Model file for the job. Use its own axes, mm. Face numbers are marked on the shaded views. A direction names the side the tool comes from. Round coordinates to 2 decimals unless told otherwise and drop trailing zeros. Order: outer loops, then holes, each group sorted by start corner. A loop starts at its lowest first (then second) coordinate and runs counter-clockwise, first axis right, second up. Notation, with made-up numbers: M 17,-28 L 48,-28 A38 cw 48,10 Z; hole C -10,35.5 d11. An arc over 180 degrees is marked long. Return JSON: item names as keys, results as strings. Group by question number.
Item 1: Pull direction Y, two halves, no side cores. Call the marked faces 4, 5 and 6: pulls with the +Y half, pulls with the -Y half, needs draft (parallel to the pull), parting line crosses it, or undercut.
Item 2: Slice it at B-B on z = 0. Write the cut outline in (x, y) (3 decimals).
Item 3: Which spindle directions (+Z, -Z, +X, -X, +Y, -Y) get a long thin tool onto all of the face, cutting with end or side? Do the marked faces 1, 2 and 3. Say none if no direction does.
Item 4: Pin check, flat tips, straight feed: pin 1 Ø3 at (y, z) = (9.5, -1) entering from +X; pin 2 Ø8 at (y, z) = (14.5, -4) entering from -X (3 decimals); pin 3 Ø5 at (y, z) = (12.5, -4.5) entering from +X; pin 4 Ø1.5 at (y, z) = (8, -1) entering from -X. Stop position of each tip, or through.
Item 5: Slice it at D-D on z = 3.5. Write the cut outline in (x, y).
Item 6: Slice it at C-C on y = 2. Write the cut outline in (x, z), then the cut area to 3 significant figures.
Item 7: Probe line 1 along Y through (x, z) = (-6.75, -5.75); line 2 along X through (y, z) = (7.75, 0). List the from-to ranges inside material, lowest first.
Item 8: Slice it at A-A on x = 0. Write the cut outline in (y, z) (3 decimals).
from build123d import *

# Parameters (mm, degrees)
SKETCH1_R           = 8.9
BOSS_EXTRUDE1_DEPTH = 1
SKETCH2_R           = 6.1
BOSS_EXTRUDE2_DEPTH = 7.6
SKETCH3_R           = 8.9
BOSS_EXTRUDE3_DEPTH = 1
SKETCH4_R           = 4.875
BOSS_EXTRUDE4_DEPTH = 7.9
CUT_EXTRUDE1_REACH  = 19.5
SKETCH5_R           = 3


with BuildPart() as part:
    # Sketch1 → Boss-Extrude1 (new body)
    with BuildSketch(Plane(origin=(0, 0, 0), x_dir=(1, 0, 0), z_dir=(0, 1, 0))):
        Circle(SKETCH1_R)
    extrude(amount=BOSS_EXTRUDE1_DEPTH)

    # Sketch2 → Boss-Extrude2 (add)
    with BuildSketch(Plane(origin=(0, 1, 0), x_dir=(1, 0, 0), z_dir=(0, 1, 0))):
        Circle(SKETCH2_R)
    extrude(amount=BOSS_EXTRUDE2_DEPTH)

    # Sketch3 → Boss-Extrude3 (add)
    with BuildSketch(Plane(origin=(0, 8.6, 0), x_dir=(1, 0, 0), z_dir=(0, 1, 0))):
        Circle(SKETCH3_R)
    extrude(amount=BOSS_EXTRUDE3_DEPTH)

    # Sketch4 → Boss-Extrude4 (add)
    with BuildSketch(Plane(origin=(0, 9.6, 0), x_dir=(1, 0, 0), z_dir=(0, 1, 0))):
        Circle(SKETCH4_R)
    extrude(amount=BOSS_EXTRUDE4_DEPTH)

    # Sketch5 → Cut-Extrude1 (cut, up to next)
    with BuildSketch(Plane(origin=(0, 17.5, 0), x_dir=(1, 0, 0), z_dir=(0, 1, 0)), mode=Mode.PRIVATE) as cut_extrude1_sk1:
        Circle(SKETCH5_R)
    cut_extrude1_tool1 = extrude(cut_extrude1_sk1.sketch, amount=-CUT_EXTRUDE1_REACH, mode=Mode.PRIVATE) & part.part
    add(cut_extrude1_tool1.solids().sort_by_distance((0, 17.5, 0))[0], mode=Mode.SUBTRACT)


solid = part.part
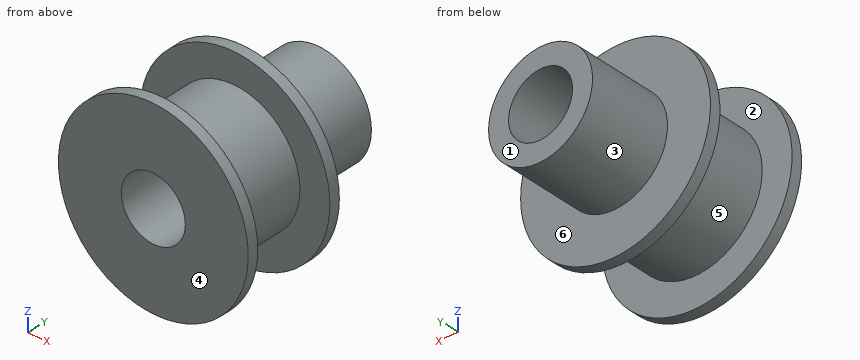
Output values:
{
 "1": {"face 4": "pulls with the -Y half", "face 5": "undercut", "face 6": "pulls with the +Y half"},
 "2": {"outline": "M -8.9,0 L -3,0 L -3,17.5 L -4.875,17.5 L -4.875,9.6 L -8.9,9.6 L -8.9,8.6 L -6.1,8.6 L -6.1,1 L -8.9,1 Z; M 3,0 L 8.9,0 L 8.9,1 L 6.1,1 L 6.1,8.6 L 8.9,8.6 L 8.9,9.6 L 4.875,9.6 L 4.875,17.5 L 3,17.5 Z"},
 "3": {"face 1": "+Z, -Z, +X, -X, +Y", "face 2": "none", "face 3": "+Y"},
 "4": {"pin 1": "x = 8.9", "pin 2": "x = -4.875", "pin 3": "x = 4.45", "pin 4": "x = -8.88"},
 "5": {"outline": "M -8.18,0 L 8.18,0 L 8.18,1 L 5,1 L 5,8.6 L 8.18,8.6 L 8.18,9.6 L 3.39,9.6 L 3.39,17.5 L -3.39,17.5 L -3.39,9.6 L -8.18,9.6 L -8.18,8.6 L -5,8.6 L -5,1 L -8.18,1 Z"},
 "6": {"outline": "C 0,0 d12.2; hole C 0,0 d6", "area": "88.6 mm²"},
 "7": {"line 1": "0 to 1, 8.6 to 9.6", "line 2": "-6.1 to -3, 3 to 6.1"},
 "8": {"outline": "M 0,-8.9 L 1,-8.9 L 1,-6.1 L 8.6,-6.1 L 8.6,-8.9 L 9.6,-8.9 L 9.6,-4.875 L 17.5,-4.875 L 17.5,-3 L 0,-3 Z; M 0,3 L 17.5,3 L 17.5,4.875 L 9.6,4.875 L 9.6,8.9 L 8.6,8.9 L 8.6,6.1 L 1,6.1 L 1,8.9 L 0,8.9 Z"}
}
